Geometry: final body of the model. Coordinates: model frame, mm. Face numbers are marked on the shaded views. A direction names the side the tool comes from. Give positions to 0.01 mm unless a question says otherwise; leave off trailing zeros. Write each loop counter-clockwise with the first axis right and the second up, starting at its lowest first coordinate (ties: lowest second). Pieces come first, ordered by that corner, then holes.
Q1. Draft query along X for the marked faces 1, 2, 3 and 4. Return one class per face: pulls with the +X half, pulls with the -X half, needs draft (parallel to the pull), parting line crosses it, or undercut.
Q2. Line query: L1, parallel to X at y = -10, z = 9.15; L2, parallel to X at y = 11, z = 4.5; L3, parallel to Z at x = 36.5, y = 9. Output: solid intervals per line, ascending.
Q3. Cut plane C-C on y = 9.5. Return the cut outline in (x, z), plus the area to 3 significant figures.
Q4. Cut plane A-A on z = 9.15. Return the cut outline in (x, y).
Q5. Cut plane B-B on x = 4. Return the cut outline in (y, z).
Q6. Reachability of the marked faces 5, 6, 7 and 8 from +Z, -Z, +X, -X, +Y, -Y: full face, straight path, thin tool, end or side. Return the list, or none.
Q7. Cut plane D-D on z = 2.75. Return the cut outline in (x, y), plus the area to 3 significant figures.
Q8. Pin query (flat end, axial travel): pin 1 (2 mm diameter, centred on x = 14.08, z = 9.15, fed in from +Y); pin 2 (0.7 mm diameter, centred on x = 10.5, z = 10, fed in from +Y); pin 3 (7.5 mm diameter, centred on x = 14.08, z = 9.15, fed in from +Y); pin 4 (1.2 mm diameter, centred on x = 12.5, z = 3, fed in from -Y). Return the tip coordinate at first contact, or that it passes through.
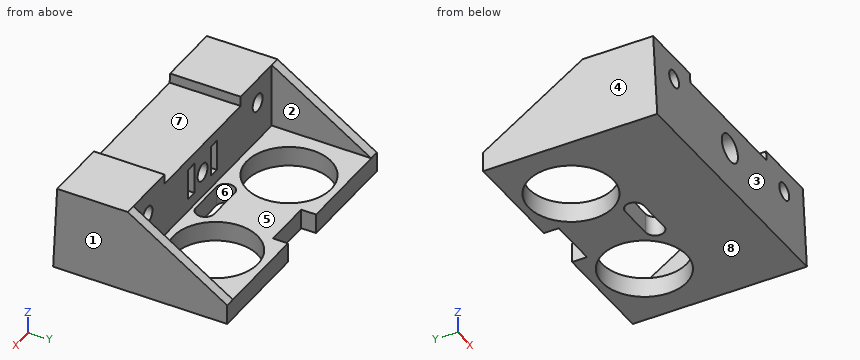
```python
from build123d import *

# Parameters (mm, degrees)
SKETCH1_R           = 8.5
BOSS_EXTRUDE1_DEPTH = 4
BOSS_EXTRUDE2_DEPTH = 13
SKETCH3_W           = 2.2
SKETCH3_H           = 6.3
CUT_EXTRUDE1_DEPTH  = 3.5
SKETCH4_R           = 1.75
CUT_EXTRUDE2_DEPTH  = 47.663174732
SKETCH6_W           = 13.5
SKETCH6_H           = 2
CUT_EXTRUDE4_DEPTH  = 47.663174732
SKETCH7_W           = 2
SKETCH7_H           = 25
BOSS_EXTRUDE3_DEPTH = 17
CUT_EXTRUDE5_DEPTH  = 72
SKETCH9_R           = 1.75
BOSS_EXTRUDE4_DEPTH = 10
SKETCH10_R          = 2.85
CUT_EXTRUDE6_DEPTH  = 12
CUT_EXTRUDE7_DEPTH  = 54


with BuildPart() as part:
    # Sketch1 → Boss-Extrude1 (new body)
    with BuildSketch(Plane.XY):
        Polygon((-10.41954023, 18.706896552), (-10.41954023, -6.293103448), (38.58045977, -6.293103448), (38.58045977, 18.706896552), (19.08045977, 18.706896552), (19.08045977, 15.706896552), (14.08045977, 15.706896552), (9.08045977, 15.706896552), (9.08045977, 18.706896552), align=None)
        with BuildLine():
            ThreePointArc((10.46545977, -0.583103448), (8.61545977, 1.266896552), (10.46545977, 3.116896552))
            Line((10.46545977, 3.116896552), (17.69545977, 3.116896552))
            ThreePointArc((17.69545977, 3.116896552), (19.54545977, 1.266896552), (17.69545977, -0.583103448))
            Line((17.69545977, -0.583103448), (10.46545977, -0.583103448))
        make_face(mode=Mode.SUBTRACT)
        with Locations((1.08045977, 8.706896552)):
            Circle(SKETCH1_R, mode=Mode.SUBTRACT)
        with Locations((27.08045977, 8.706896552)):
            Circle(SKETCH1_R, mode=Mode.SUBTRACT)
    extrude(amount=BOSS_EXTRUDE1_DEPTH)

    # Sketch2 → Boss-Extrude2 (add)
    with BuildSketch(Plane.XY.offset(4)):
        Polygon((14.08045977, -1.293103448), (38.58045977, -1.293103448), (38.58045977, -6.293103448), (-10.41954023, -6.293103448), (-10.41954023, -1.293103448), align=None)
    extrude(amount=BOSS_EXTRUDE2_DEPTH)

    # Sketch3 → Cut-Extrude1 (cut)
    with BuildSketch(Plane(origin=(0, -1.293103448, 0), x_dir=(1, 0, 0), z_dir=(0, 1, 0))):
        with Locations((10.08045977, -9.65)):
            Rectangle(SKETCH3_W, SKETCH3_H)
        with Locations((18.08045977, -9.65)):
            Rectangle(SKETCH3_W, SKETCH3_H)
    extrude(amount=-CUT_EXTRUDE1_DEPTH, mode=Mode.SUBTRACT)

    # Sketch4 → Cut-Extrude2 (cut, through all)
    with BuildSketch(Plane(origin=(0, -1.293103448, 0), x_dir=(1, 0, 0), z_dir=(0, 1, 0))):
        with Locations(Location((14.08045977, -9.15, 0), (0, 0, 270))):
            Circle(SKETCH4_R)
        with Locations(Location((33.58045977, -12, 0), (0, 0, 270))):
            Circle(SKETCH4_R)
        with Locations(Location((-5.41954023, -12, 0), (0, 0, 90))):
            Circle(SKETCH4_R)
    extrude(amount=-CUT_EXTRUDE2_DEPTH, mode=Mode.SUBTRACT)

    # Sketch6 → Cut-Extrude4 (cut, through all)
    with BuildSketch(Plane(origin=(0, -1.293103448, 0), x_dir=(1, 0, 0), z_dir=(0, 1, 0))):
        with Locations((7.33045977, -16)):
            Rectangle(SKETCH6_W, SKETCH6_H)
        with Locations((20.83045977, -16)):
            Rectangle(SKETCH6_W, SKETCH6_H)
    extrude(amount=-CUT_EXTRUDE4_DEPTH, mode=Mode.SUBTRACT)

    # Sketch7 → Boss-Extrude3 (add)
    with BuildSketch(Plane(origin=(0, 0, 0), x_dir=(-1, 0, 0), z_dir=(0, 0, -1))):
        with Locations((-39.58045977, 6.206896552)):
            Rectangle(SKETCH7_W, SKETCH7_H)
        with Locations((11.41954023, 6.206896552)):
            Rectangle(SKETCH7_W, SKETCH7_H)
    extrude(amount=-BOSS_EXTRUDE3_DEPTH)

    # Sketch8 → Cut-Extrude5 (cut)
    with BuildSketch(Plane(origin=(40.58045977, 0, 0), x_dir=(0, 0, -1), z_dir=(1, 0, 0))):
        Polygon((-4, 18.706896552), (-17, -1.293103448), (-17, 18.706896552), align=None)
    extrude(amount=-CUT_EXTRUDE5_DEPTH, mode=Mode.SUBTRACT)

    # Sketch9 → Boss-Extrude4 (add)
    with BuildSketch(Plane(origin=(0, -6.293103448, 0), x_dir=(-1, 0, 0), z_dir=(0, -1, 0))):
        Polygon((-40.58045977, 0), (-40.58045977, -17), (-27.58045977, -17), (-27.58045977, -15), (-0.58045977, -15), (-0.58045977, -17), (12.41954023, -17), (12.41954023, 0), align=None)
        with Locations(Location((5.41954023, -12, 0), (0, 0, 90))):
            Circle(SKETCH9_R, mode=Mode.SUBTRACT)
        with Locations(Location((-14.08045977, -9.15, 0), (0, 0, 270))):
            Circle(SKETCH9_R, mode=Mode.SUBTRACT)
        with Locations(Location((-33.58045977, -12, 0), (0, 0, 270))):
            Circle(SKETCH9_R, mode=Mode.SUBTRACT)
    extrude(amount=BOSS_EXTRUDE4_DEPTH)

    # Sketch10 → Cut-Extrude6 (cut)
    with BuildSketch(Plane(origin=(0, -16.293103448, 0), x_dir=(-1, 0, 0), z_dir=(0, -1, 0))):
        with Locations(Location((-14.08045977, -9.15, 0), (0, 0, 90))):
            Circle(SKETCH10_R)
    extrude(amount=-CUT_EXTRUDE6_DEPTH, mode=Mode.SUBTRACT)

    # Sketch11 → Cut-Extrude7 (cut)
    with BuildSketch(Plane.ZY.offset(12.41954023)):
        Polygon((17, -16.293103448), (17, -15.482482603), (0, -16.293103448), align=None)
    extrude(amount=-CUT_EXTRUDE7_DEPTH, mode=Mode.SUBTRACT)


solid = part.part
```
Data:
1. face 1: pulls with the +X half
1. face 2: undercut
1. face 3: needs draft
1. face 4: pulls with the -X half
2. L1: x = -12.42 to 11.23, 16.93 to 40.58
2. L2: x = -12.42 to -10.42, 38.58 to 40.58
2. L3: z = 0 to 4
3. outline: (-12.42, 0) - (-7.38, 0) - (-7.38, 4) - (-10.42, 4) - (-10.42, 9.98) - (-12.42, 9.98) - close; (9.54, 0) - (18.62, 0) - (18.62, 4) - (9.54, 4) - close; (35.54, 0) - (40.58, 0) - (40.58, 9.98) - (38.58, 9.98) - (38.58, 4) - (35.54, 4) - close
3. area: 101 mm2
4. outline: (-12.42, -15.86) - (11.23, -15.86) - (11.23, -4.29) - (12.33, -4.29) - (12.33, -1.29) - (11.18, -1.29) - (11.18, -4.79) - (8.98, -4.79) - (8.98, -1.29) - (-10.42, -1.29) - (-10.42, 10.78) - (-12.42, 10.78) - close; (15.83, -4.29) - (16.93, -4.29) - (16.93, -15.86) - (40.58, -15.86) - (40.58, 10.78) - (38.58, 10.78) - (38.58, -1.29) - (19.18, -1.29) - (19.18, -4.79) - (16.98, -4.79) - (16.98, -1.29) - (15.83, -1.29) - close
5. outline: (-16.29, 0) - (0.72, 0) - (0.72, 4) - (-1.29, 4) - (-1.29, 15) - (-15.58, 15) - close; (16.69, 0) - (18.71, 0) - (18.71, 4) - (16.69, 4) - close
6. face 5: +Z, +Y
6. face 6: +Z, -Z
6. face 7: +Z, +Y, -Y
6. face 8: -Z, +X, -X, +Y, -Y
7. outline: (-12.42, -16.16) - (40.58, -16.16) - (40.58, 18.71) - (19.08, 18.71) - (19.08, 15.71) - (9.08, 15.71) - (9.08, 18.71) - (-12.42, 18.71) - close; hole circle Ø17 at (1.08, 8.71); hole (10.47, -0.58) - (17.7, -0.58) arc R1.85 ccw to (17.7, 3.12) - (10.47, 3.12) arc R1.85 ccw to start; hole circle Ø17 at (27.08, 8.71)
7. area: 1,330 mm2
8. pin 1: passes through
8. pin 2: stops at y = -4.79
8. pin 3: stops at y = -1.29
8. pin 4: stops at y = -16.18
